Autodesk Fusion 360 part; units mm, degrees
sketch "Sketch1" plane through (0, 0, 0) normal (0, 0, 1) x (1, 0, 0)
  line L0 (39.5, 28) -> (-39.5, 28)
  line L1 (-39.5, 28) -> (-39.5, -28)
  line L2 (-39.5, -28) -> (39.5, -28)
  line L3 (39.5, -28) -> (39.5, 28)
  line L4 (39.5, 28) -> (-39.5, -28) construction
  line L5 (-39.5, 28) -> (39.5, -28) construction
  dimension "d1" = 79
  dimension "d2" = 56
extrude "Extrude1" add sketch "Sketch1" along normal blind 22.5
sketch "Sketch2" plane through (0, 0, 22.5) normal (0, 0, 1) x (-1, 0, 0)
  line L0 (-39.5, 28) -> (-39.5, -28)
  line L1 (-39.5, -28) -> (39.5, -28)
  line L2 (39.5, -28) -> (39.5, 28)
  line L3 (39.5, 28) -> (-39.5, 28)
  line L4 (-36.5, -25) -> (36.5, -25)
  line L5 (36.5, -25) -> (36.5, 25)
  line L6 (36.5, 25) -> (-36.5, 25)
  line L7 (-36.5, 25) -> (-36.5, -25)
  line L8 (-36.5, -25) -> (36.5, 25) construction
  line L9 (36.5, -25) -> (-36.5, 25) construction
  dimension "d5" = 73
  dimension "d6" = 50
extrude "Extrude2" cut sketch "Sketch2" against normal blind 19.5 contours L4 L5 L6 L7
sketch "Sketch3" plane through (0, 0, 0) normal (0, 0, -1) x (1, 0, 0)
  line L0 (39.5, -28) -> (39.5, 28)
  line L1 (39.5, 28) -> (-39.5, 28)
  line L2 (-39.5, 28) -> (-39.5, -28)
  line L3 (-39.5, -28) -> (39.5, -28)
  line L4 (33.25, 21.75) -> (-33.25, 21.75)
  line L5 (-33.25, 21.75) -> (-33.25, -21.75)
  line L6 (-33.25, -21.75) -> (33.25, -21.75)
  line L7 (33.25, -21.75) -> (33.25, 21.75)
  line L8 (33.25, 21.75) -> (-33.25, -21.75) construction
  line L9 (-33.25, 21.75) -> (33.25, -21.75) construction
  dimension "d9" = 66.5
  dimension "d10" = 43.5
sketch "Sketch4" plane through (0, 0, 0) normal (0, 0, -1) x (1, 0, 0)
extrude "Extrude3" cut sketch "Sketch3" against normal blind 3 contours L4 L5 L6 L7
sketch "Sketch5" plane through (0, 0, 3) normal (0, 0, 1) x (-1, 0, 0)
  line L0 (-33.25, 21.75) -> (33.25, 21.75)
  line L1 (33.25, 21.75) -> (33.25, -21.75)
  line L2 (33.25, -21.75) -> (-33.25, -21.75)
  line L3 (-33.25, -21.75) -> (-33.25, 21.75)
  line L4 (-36.5, 25) -> (-36.5, -25)
  line L5 (-36.5, -25) -> (36.5, -25)
  line L6 (36.5, -25) -> (36.5, 25)
  line L7 (36.5, 25) -> (-36.5, 25)
  circle A0 centre (34.875, -23.375) radius 1.5
  dimension "d13" = 3
  dimension "d14" = 1.625
  dimension "d15" = 1.625
sketch "Sketch6" plane through (0, 0, 3) normal (0, 0, 1) x (-1, 0, 0)
  circle A0 centre (-34.875, -23.375) radius 1.5
  line L0 (-36.5, -25) -> (36.5, -25)
  line L1 (-36.5, 25) -> (-36.5, -25)
  circle A1 centre (-34.875, 23.375) radius 1.5
  line L2 (36.5, 25) -> (-36.5, 25)
  circle A2 centre (34.875, 23.375) radius 1.5
  line L3 (36.5, -25) -> (36.5, 25)
  dimension "d16" = 3
  dimension "d17" = 1.625
  dimension "d18" = 1.625
  dimension "d19" = 3
  dimension "d20" = 1.625
  dimension "d21" = 1.625
  dimension "d25" = 3
  dimension "d26" = 1.625
  dimension "d27" = 1.625
sketch "Sketch7" plane through (0, 0, 3) normal (0, 0, 1) x (-1, 0, 0)
  circle A0 centre (34.875, 23.375) radius 1.55
  line L0 (36.5, 25) -> (-36.5, 25)
  line L1 (36.5, -25) -> (36.5, 25)
  dimension "d22" = 3.1
  dimension "d23" = 1.625
  dimension "d24" = 1.625
extrude "Extrude4" add sketch "Sketch5" sketch "Sketch7" sketch "Sketch6" along normal blind 4 contours A0 of sketch 2 of sketch 3 contours A0 | A1
sketch "Sketch8" plane through (0, -28, 0) normal (0, -1, 0) x (1, 0, 0)
  line L0 (-39.5, 0) -> (39.5, 0)
  line L1 (39.5, 0) -> (39.5, 22.5)
  line L2 (39.5, 22.5) -> (-39.5, 22.5)
  line L3 (-39.5, 22.5) -> (-39.5, 0)
  line L4 (31.5, 15) -> (-31.5, 15)
  line L5 (-31.5, 15) -> (-31.5, 5)
  line L6 (-31.5, 5) -> (31.5, 5)
  line L7 (31.5, 5) -> (31.5, 15)
  line L8 (31.5, 15) -> (-31.5, 5) construction
  line L9 (-31.5, 15) -> (31.5, 5) construction
  point P0 (0, 10)
  dimension "d30" = 63
  dimension "d31" = 10
  dimension "d33" = 15
extrude "Extrude5" cut sketch "Sketch8" against normal blind 3 contours L4 L5 L6 L7
sketch "Sketch9" plane through (0, 28, 0) normal (0, 1, 0) x (-1, 0, 0)
  line L0 (-39.5, 0) -> (39.5, 0)
  line L1 (39.5, 0) -> (39.5, 22.5)
  line L2 (39.5, 22.5) -> (-39.5, 22.5)
  line L3 (-39.5, 22.5) -> (-39.5, 0)
  line L4 (31.5, 15) -> (1.5, 15)
  line L5 (1.5, 15) -> (1.5, 5)
  line L6 (1.5, 5) -> (31.5, 5)
  line L7 (31.5, 5) -> (31.5, 15)
  line L8 (31.5, 15) -> (1.5, 5) construction
  line L9 (1.5, 15) -> (31.5, 5) construction
  point P0 (16.5, 10)
  dimension "d36" = 30
  dimension "d37" = 10
  dimension "d38" = 8
  dimension "d39" = 15
extrude "Extrude6" cut sketch "Sketch9" against normal blind 3 contours L4 L5 L6 L7
sketch "Sketch11" plane through (0, 0, 22.5) normal (0, 0, 1) x (-1, 0, 0)
  line L0 (36.5, -25) -> (-36.5, -25)
  line L1 (-36.5, -25) -> (-36.5, 25)
  line L2 (-36.5, 25) -> (36.5, 25)
  line L3 (36.5, 25) -> (36.5, -25)
  line L4 (-39.5, 28) -> (-39.5, -28)
  line L5 (-39.5, -28) -> (39.5, -28)
  line L6 (39.5, -28) -> (39.5, 28)
  line L7 (39.5, 28) -> (-39.5, 28)
  circle A0 centre (37.375, -25.875) radius 1
  circle A1 centre (37.375, 25.875) radius 1
  circle A2 centre (-37.375, 25.875) radius 1
  circle A3 centre (-37.375, -25.875) radius 1
  dimension "d56" = 2
  dimension "d57" = 2
  dimension "d58" = 2
  dimension "d59" = 2
  dimension "d60" = 2.125
  dimension "d61" = 2.125
  dimension "d62" = 2.125
  dimension "d63" = 2.125
  dimension "d64" = 2.125
  dimension "d65" = 2.125
  dimension "d66" = 2.125
  dimension "d67" = 2.125
hole "Hole1" at (-37.375, 25.875, 22.5) at (37.375, 25.875, 22.5) at (37.375, -25.875, 22.5) at (-37.375, -25.875, 22.5) direction (0, 0, -1) diameter 1.6256 depth 5 tip angle 180
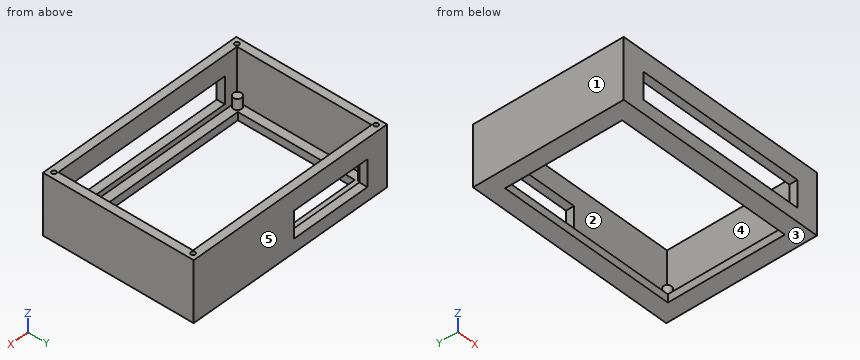
Read the model definition and answer for the solid it produces. Units are mm, in the model's axes. Face numbers are marked on the shaded views. A direction names the side the tool comes from. Give positions to 0.01 mm unless a question says otherwise; leave off trailing zeros. Write each loop counter-clockwise with the first axis right and the second up, starting at its lowest first coordinate (ties: lowest second). Pieces come first, ordered by that corner, then holes. Notation, with made-up numbers: (87.5, -5.75) -> (111.5, -5.75) arc R9 ccw to (111.5, 7.25) -> close; hole circle Ø8 at (-39.5, -16). An arc over 180 degrees is marked (long way). Answer in a Markdown table with one row per item.
1) Determine the mould class of the marked faces 1, 2 and 3 for opening direction X: released by +X, released by -X, zero draft, split by the parting line, or undercut.
Results list:
| item | result |
|---|---|
| face 1 | released by -X |
| face 2 | undercut |
| face 3 | zero draft |
2) Each of these flat-tipped pins is pushed along its axis until it touches: pin 1 Ø10 at (x, y) = (15, -12) entering from +Z; pin 2 Ø0.9 at (x, y) = (35, 23) entering from +Z; pin 3 Ø0.8 at (x, y) = (-37.5, -26) entering from +Z. Where does it stop, or does it pass through?
Results list:
| item | result |
|---|---|
| pin 1 | through |
| pin 2 | z = 7 |
| pin 3 | z = 17.5 |
3) Section D-D on x = -23 is taken. Give the vertices of the cut face in (y, z).
Results list:
| item | result |
|---|---|
| outline | (-28, 0) -> (-21.75, 0) -> (-21.75, 3) -> (-25, 3) -> (-25, 5) -> (-28, 5) -> close; (-28, 15) -> (-25, 15) -> (-25, 22.5) -> (-28, 22.5) -> close; (21.75, 0) -> (28, 0) -> (28, 5) -> (25, 5) -> (25, 3) -> (21.75, 3) -> close; (25, 15) -> (28, 15) -> (28, 22.5) -> (25, 22.5) -> close |
4) Section B-B on y = 3 is taken. Give the vertices of the cut face in (x, z).
Results list:
| item | result |
|---|---|
| outline | (-39.5, 0) -> (-33.25, 0) -> (-33.25, 3) -> (-36.5, 3) -> (-36.5, 22.5) -> (-39.5, 22.5) -> close; (33.25, 0) -> (39.5, 0) -> (39.5, 22.5) -> (36.5, 22.5) -> (36.5, 3) -> (33.25, 3) -> close |
5) A tool of negligible diameter and unlimited length cuts with its end or side. For the marked faces 4 and 5, from which of +Z, -Z, +X, -X, +Y, -Y can it reach the whole face along a straight path? Write none if from no direction.
Results list:
| item | result |
|---|---|
| face 4 | +Z |
| face 5 | +Z, -Z, +X, -X, +Y |
6) Section C-C on z = 8 is taken. Give the vertices of the cut face in (x, y), plus the area to 3 significant figures.
Results list:
| item | result |
|---|---|
| outline | (-39.5, -28) -> (-31.5, -28) -> (-31.5, -25) -> (-36.5, -25) -> (-36.5, 25) -> (-31.5, 25) -> (-31.5, 28) -> (-39.5, 28) -> close; (-1.5, 25) -> (36.5, 25) -> (36.5, -25) -> (31.5, -25) -> (31.5, -28) -> (39.5, -28) -> (39.5, 28) -> (-1.5, 28) -> close |
| area | 495 mm^2 |
7) Straight lines are drawn through the part: line 1 (Y direction, x = 32.5, z = 4.5); line 2 (X direction, y = 5, z = 11.5); line 3 (Y direction, x = -10, z = 2.25). For each, find the intervals that lie inside material, in ascending order. Write a range as [from, to].
Results list:
| item | result |
|---|---|
| line 1 | [-28, -25], [25, 28] |
| line 2 | [-39.5, -36.5], [36.5, 39.5] |
| line 3 | [-28, -21.75], [21.75, 28] |
8) Section A-A on x = 18.5 is taken. Give the vertices of the cut face in (y, z), plus the area to 4 significant figures.
Results list:
| item | result |
|---|---|
| outline | (-28, 0) -> (-21.75, 0) -> (-21.75, 3) -> (-25, 3) -> (-25, 5) -> (-28, 5) -> close; (-28, 15) -> (-25, 15) -> (-25, 22.5) -> (-28, 22.5) -> close; (21.75, 0) -> (28, 0) -> (28, 22.5) -> (25, 22.5) -> (25, 3) -> (21.75, 3) -> close |
| area | 124.5 mm^2 |
